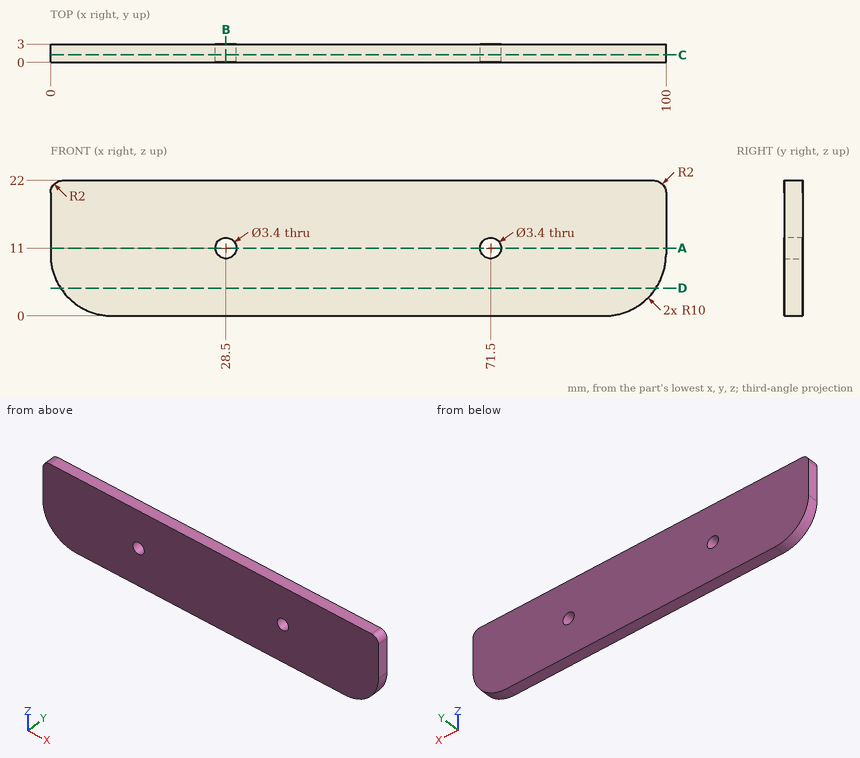
Geometry check sheet. Reference: drawing and pictorial views, mm from the part's lowest x, y, z. Give positions to 0.01 mm unless a question says otherwise; leave off trailing zeros. Order: outer loops, then holes, each group sorted by start corner. A loop starts at its lowest first (then second) coordinate and runs counter-clockwise, first axis right, second up. Notation, with made-up numbers: M 50.5,55 L 86.5,55 A24 ccw 86.5,90 Z; hole C -13,-9.5 d8. An arc over 180 degrees is marked long. Answer as CSV lines item,"result". Start each with the question number.
Item 1: Gauge pin test, flat ends, axial feed: P1, Ø1, axis at x = 61.5, z = 17, coming from the -Y side; P2, Ø2, axis at x = 28.5, z = 11, coming from the -Y side. Record the tip position at first contact, or that the pin passes through.
Item 2: Cross-section at A-A on z = 11. Enter the section's corners in (x, y), plus the area to 3 significant figures.
Item 3: Cross-section at B-B on x = 28.5. Enter the section's corners in (y, z).
Item 4: Thickness scan on line 1 (X direction, y = 1.3, z = 11); line 2 (Z direction, x = 71.5, y = 0.85); line 3 (X direction, y = 0.9, z = 11.5). Record the ranges inside material, lowest first. Write a range as [from, to].
Item 5: Cross-section at D-D on z = 4.5. Enter the section's corners in (x, y), plus the area to 3 significant figures.
Item 6: Cross-section at C-C on y = 1.25. Enter the section's corners in (x, z), plus the area to 3 significant figures.
Established:
1,P1,"stops at y = 0"
1,P2,"passes through"
2,outline,"M 0,0 L 26.8,0 L 26.8,3 L 0,3 Z; M 30.2,0 L 69.8,0 L 69.8,3 L 30.2,3 Z; M 73.2,0 L 100,0 L 100,3 L 73.2,3 Z"
2,area,"280 mm^2"
3,outline,"M 0,0 L 3,0 L 3,9.3 L 0,9.3 Z; M 0,12.7 L 3,12.7 L 3,22 L 0,22 Z"
4,line 1,"x = [0, 26.8], [30.2, 69.8], [73.2, 100]"
4,line 2,"z = [0, 9.3], [12.7, 22]"
4,line 3,"x = [0, 26.88], [30.12, 69.88], [73.12, 100]"
5,outline,"M 1.65,0 L 98.35,0 L 98.35,3 L 1.65,3 Z"
5,area,"290 mm^2"
6,outline,"M 0,10 A10 ccw 10,0 L 90,0 A10 ccw 100,10 L 100,20 A2 ccw 98,22 L 2,22 A2 ccw 0,20 Z; hole C 28.5,11 d3.4; hole C 71.5,11 d3.4"
6,area,"2,140 mm^2"
